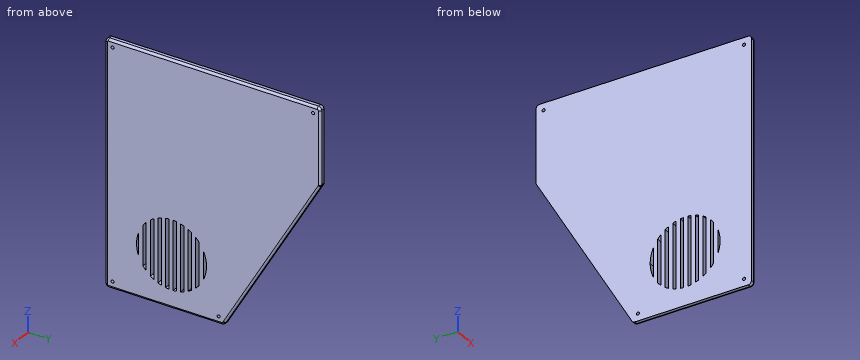
```python
from build123d import *

# Parameters (mm, degrees)
SKETCH2_R           = 1.4
SKETCH2_R_2         = 1.414097505
BOSS_EXTRUDE2_DEPTH = 5
CUT_EXTRUDE1_DEPTH  = 5
FILLET4_R           = 2


with BuildPart() as part:
    # Sketch2 → Boss-Extrude2 (new body)
    with BuildSketch(Plane(origin=(0, 0, 0), x_dir=(0, 0, -1), z_dir=(1, 0, 0))):
        with BuildLine():
            Line((-137.05346623, 114.041314814), (-137.05346623, -79.958685186))
            ThreePointArc((-137.05346623, -79.958685186), (-136.174786573, -82.08000553), (-134.05346623, -82.958685186))
            Line((-134.05346623, -82.958685186), (89.94653377, -82.958685186))
            ThreePointArc((89.94653377, -82.958685186), (92.067854114, -82.08000553), (92.94653377, -79.958685186))
            Line((92.94653377, -79.958685186), (92.94653377, 25.368162352))
            ThreePointArc((92.94653377, 25.368162352), (92.541535124, 26.8734756), (91.435888454, 27.97235563))
            Line((91.435888454, 27.97235563), (90.428791577, 28.548320734))
            Line((90.428791577, 28.548320734), (-63.7480103, 116.646068127))
            ThreePointArc((-63.7480103, 116.646068127), (-64.466404774, 116.940819939), (-65.236385313, 117.041314814))
            Line((-65.236385313, 117.041314814), (-134.05346623, 117.041314814))
            ThreePointArc((-134.05346623, 117.041314814), (-136.174786573, 116.162635157), (-137.05346623, 114.041314814))
        make_face()
        with Locations((-130.402194721, 110.164268622)):
            Circle(SKETCH2_R, mode=Mode.SUBTRACT)
        with Locations((-130.378834203, -76.102450402)):
            Circle(SKETCH2_R, mode=Mode.SUBTRACT)
        with Locations((86.178766817, -76.190918233)):
            Circle(SKETCH2_R_2, mode=Mode.SUBTRACT)
        with Locations((86.178766817, 22.440231448)):
            Circle(SKETCH2_R, mode=Mode.SUBTRACT)
    extrude(amount=BOSS_EXTRUDE2_DEPTH)

    # Sketch3 → Cut-Extrude1 (cut)
    with BuildSketch(Plane(origin=(5, 0, 0), x_dir=(0, 0, -1), z_dir=(1, 0, 0))):
        with BuildLine():
            ThreePointArc((43.568031387, 11.142105509), (36.585911365, 10.383246006), (29.92984969, 8.142105509))
            Line((29.92984969, 8.142105509), (57.206213084, 8.142105509))
            ThreePointArc((57.206213084, 8.142105509), (50.550151409, 10.383246006), (43.568031387, 11.142105509))
        make_face()
        with BuildLine():
            ThreePointArc((23.418589707, 4.142105509), (21.715728373, 2.69884787), (20.115952588, 1.142105509))
            Line((20.115952588, 1.142105509), (67.020110186, 1.142105509))
            ThreePointArc((67.020110186, 1.142105509), (65.420334401, 2.69884787), (63.717473066, 4.142105509))
            Line((63.717473066, 4.142105509), (23.418589707, 4.142105509))
        make_face()
        with BuildLine():
            Line((70.288809819, -2.857894491), (16.847252955, -2.857894491))
            ThreePointArc((16.847252955, -2.857894491), (15.884118126, -4.332885047), (15.002317673, -5.857894491))
            Line((15.002317673, -5.857894491), (72.133745101, -5.857894491))
            ThreePointArc((72.133745101, -5.857894491), (71.251944648, -4.332885047), (70.288809819, -2.857894491))
        make_face()
        with BuildLine():
            Line((73.965399694, -9.857894491), (13.17066308, -9.857894491))
            ThreePointArc((13.17066308, -9.857894491), (12.648553826, -11.346106069), (12.199257104, -12.857894491))
            Line((12.199257104, -12.857894491), (74.93680567, -12.857894491))
            ThreePointArc((74.93680567, -12.857894491), (74.487508947, -11.346106069), (73.965399694, -9.857894491))
        make_face()
        with BuildLine():
            Line((75.754985266, -16.857894491), (11.381077508, -16.857894491))
            ThreePointArc((11.381077508, -16.857894491), (11.207088544, -18.354666502), (11.102665225, -19.857894491))
            Line((11.102665225, -19.857894491), (76.033397548, -19.857894491))
            ThreePointArc((76.033397548, -19.857894491), (75.928974229, -18.354666502), (75.754985266, -16.857894491))
        make_face()
        with BuildLine():
            Line((75.971734879, -23.857894491), (11.164327895, -23.857894491))
            ThreePointArc((11.164327895, -23.857894491), (11.315662222, -25.362227549), (11.536796631, -26.857894491))
            Line((11.536796631, -26.857894491), (75.599266143, -26.857894491))
            ThreePointArc((75.599266143, -26.857894491), (75.820400552, -25.362227549), (75.971734879, -23.857894491))
        make_face()
        with BuildLine():
            Line((74.648571923, -30.857894491), (12.487490851, -30.857894491))
            ThreePointArc((12.487490851, -30.857894491), (12.990946698, -32.371154315), (13.568031387, -33.857894491))
            Line((13.568031387, -33.857894491), (73.568031387, -33.857894491))
            ThreePointArc((73.568031387, -33.857894491), (74.145116075, -32.371154315), (74.648571923, -30.857894491))
        make_face()
        with BuildLine():
            Line((71.568031387, -37.857894491), (15.568031387, -37.857894491))
            ThreePointArc((15.568031387, -37.857894491), (16.526396821, -39.385650868), (17.568031387, -40.857894491))
            Line((17.568031387, -40.857894491), (69.568031387, -40.857894491))
            ThreePointArc((69.568031387, -40.857894491), (70.609665953, -39.385650868), (71.568031387, -37.857894491))
        make_face()
        with BuildLine():
            Line((66.017975707, -44.857894491), (21.118087066, -44.857894491))
            ThreePointArc((21.118087066, -44.857894491), (22.881161375, -46.423875603), (24.753143665, -47.857894491))
            Line((24.753143665, -47.857894491), (62.382919109, -47.857894491))
            ThreePointArc((62.382919109, -47.857894491), (64.254901399, -46.423875603), (66.017975707, -44.857894491))
        make_face()
        with BuildLine():
            Line((54.793003547, -51.857894491), (32.343059226, -51.857894491))
            ThreePointArc((32.343059226, -51.857894491), (43.568031387, -53.857894491), (54.793003547, -51.857894491))
        make_face()
    extrude(amount=-CUT_EXTRUDE1_DEPTH, mode=Mode.SUBTRACT)

    # Fillet4
    fillet4_edges = [part.edges().sort_by_distance(p)[0] for p in [
        (5, -82.08000553, 136.174786573),
        (5, -82.958685186, 22.05346623),
        (5, -82.08000553, -92.067854114),
        (5, -27.295261417, -92.94653377),
        (5, 26.8734756, -92.541535124),
        (5, 28.260338182, -90.932340015),
        (5, 72.59719443, -13.340390638),
        (5, 116.940819939, 64.466404774),
        (5, 117.041314814, 99.644925771),
        (5, 116.162635157, 136.174786573),
        (5, 17.041314814, 137.05346623),
    ]]
    fillet(fillet4_edges, radius=FILLET4_R)


solid = part.part
```
Part model, mm, in its own coordinate system. Round coordinates to 2 decimals unless told otherwise and drop trailing zeros. Use a Markdown table: item, result.
1) Probe line 1 (Z direction, x = 3.2, y = -29.5); line 2 (Y direction, x = 3.3, z = 106); line 3 (Y direction, x = 2.7, z = -75). List the from-to ranges inside material, lowest first. Write a range as [from, to].
The answers:
| item | result |
|---|---|
| line 1 | z = [-92.94, 137.04] |
| line 2 | y = [-82.94, 117.02] |
| line 3 | y = [-82.96, -26.86], [-23.86, -19.86], [-16.86, 37.36] |
2) Cut at A-A, the plane x = 4.25. State how many separate pieces and enclosed holes the cut face has, and give its area (3 significant figures).
The answers:
| item | result |
|---|---|
| separate pieces | 1 |
| enclosed holes | 14 |
| area | 37,100 mm2 |
3) Drop flat-ended pins along their axis: pin 1 Ø1.5 at (x, z) = (2.5, -40.5) entering from +Y; pin 2 Ø1 at (x, z) = (4.5, -64.5) entering from -Y; pin 3 Ø2.5 at (x, z) = (1.5, -57.5) entering from +Y. Give the stop position or say it passes through.
The answers:
| item | result |
|---|---|
| pin 1 | stops at y = 57.51 |
| pin 2 | stops at y = -82.69 |
| pin 3 | stops at y = 48.08 |
